Design review of the part built by this model. Coordinates are the model's own, in mm. A direction names the side the tool comes from. Coordinates: 2 decimals unless noted, no trailing zeros. Loops run counter-clockwise (first coordinate to the right, second up) from the corner with the lowest first, then second, coordinate; pieces in that order, holes last. Notation, with made-up numbers: (24.25, 73) -> (81.25, 73) arc R22 ccw to (81.25, 104) -> close; hole circle Ø10 at (22, 17). An arc over 180 degrees is marked (long way). One line per item, written item: value. Start each with the question number.
1. Add section C-C on z = 8.5. Write out the cut boundary in (x, y).
2. For probe 1 along X at (y, z) = (-72.5, 8.5); probe 2 along X at (y, z) = (-45.5, 58.5); probe 3 along X at (y, z) = (-45, 65), list the stretches that pass through material, from the lowest coordinate up.
3. Add section D-D on z = 55. Write out the cut boundary in (x, y), plus the area to 3 significant figures.
4. Draft analysis for pull direction X (two halves, no side actions). For faces 6 (the flat face through (-48.26, -76, 30)), 7 (the flat face through (-139, -67.31, 24)), 8 (the flat face through (157.48, -1, 24)), state which applies: pulls with the +X half, pulls with the -X half, needs draft (parallel to the pull), parting line crosses it, or undercut.
5. Insertion check: pin 1 (4 mm diameter, centred on y = -16.5, z = 70.5, fed in from +X); pin 2 (18 mm diameter, centred on x = -139, z = 17.5, fed in from +Y); pin 3 (8 mm diameter, centred on x = -105, y = 64, fed in from +Z). Each pin has a flat end and moves straight along its axis. Give the tip position at first contact, or say it passes through.
6. Add section A-A on x = -68.5. Write out the cut boundary in (y, z), plus the area to 3 significant figures.
7. Add section B-B on y = -22. Write out the cut boundary in (x, z).
8. Machinability: for faces 1 (the flat face through (-48.26, 75, 30)), 2 (the flat face through (140, 67.31, 24)), 3 (the flat face through (121.92, -1, 50)), 4 (the flat face through (-139, 67.31, 24)), 5 (the flat face through (-140, 1, 48.26)), which of the approach directions +Z, -Z, +X, -X, +Y, -Y give a long, thin tool a straight path to every point of the face, cutting with its end or side? Answer none if there is none.
```python
from build123d import *

# Parameters (mm, degrees)
F1_DEPTH   = 48.26
F2_W       = 35.56
F2_H       = 15.24
F3_DEPTH   = 25.4
F4_DEPTH   = 73.66
F5_START   = -73.66
F4_FACE_W  = 15.24
F4_FACE_H  = 25.4
F5_DEPTH   = 78.74
F6_DEPTH   = 22.86
F7_START   = 96.52
F6_FACE_W  = 15.24
F6_FACE_H  = 48.26
F7_DEPTH   = 73.66
F9_W       = 157.48
F9_H       = 67.31
F10_DEPTH  = 48.26
F11_W      = 35.56
F11_H      = 48.26
F12_DEPTH  = 16.51
F13_DEPTH  = 73.66
F14_START  = -73.66
F13_FACE_W = 16.51
F13_FACE_H = 48.26
F14_DEPTH  = 78.74
F18_DEPTH  = 12.7
F19_W      = 35.56
F19_H      = 134.62
F20_DEPTH  = 12.7
F22_DEPTH  = 13.97


with BuildPart() as f1:
    # F0 (on Top) → F1 (new body)
    with BuildSketch(Plane.XY):
        Polygon((0, 134.62), (0, 0), (314.96, 0), (314.96, 134.62), (35.56, 134.62), align=None)
    extrude(amount=F1_DEPTH)

    # F2 (on face) → F3 (join)
    with BuildSketch(Plane.XY.offset(48.26)):
        with Locations((17.78, 142.24)):
            Rectangle(F2_W, F2_H)
    extrude(amount=-F3_DEPTH)

    # F4 (add): a face of the model
    f4_faces = [f1.faces().sort_by_distance(p)[0] for p in [
        (35.56, 142.24, 35.56),
    ]]
    extrude(f4_faces, amount=F4_DEPTH)

    # F4_face (on face) → F5 (cut)
    with BuildSketch(Plane(origin=(109.22, 142.24, 35.56), x_dir=(0, 1, 0), z_dir=(1, 0, 0)).offset(F5_START)):
        Rectangle(F4_FACE_W, F4_FACE_H)
    extrude(amount=-F5_DEPTH, mode=Mode.SUBTRACT)

    # F6 (add): a face of the model
    f6_faces = [f1.faces().sort_by_distance(p)[0] for p in [
        (72.39, 142.24, 22.86),
    ]]
    extrude(f6_faces, amount=F6_DEPTH)

    # F6_face (on face) → F7 (join)
    with BuildSketch(Plane(origin=(109.22, 142.24, 24.13), x_dir=(0, 1, 0), z_dir=(1, 0, 0)).offset(F7_START)):
        Rectangle(F6_FACE_W, F6_FACE_H)
    extrude(amount=F7_DEPTH)


with BuildPart() as f10:
    # F9 (on Top) → F10 (new body)
    with BuildSketch(Plane.XY):
        with Locations((78.74, 33.655)):
            Rectangle(F9_W, F9_H)
    extrude(amount=F10_DEPTH)

    # F11 (on face) → F12 (join)
    with BuildSketch(Plane(origin=(0, 67.31, 0), x_dir=(-1, 0, 0), z_dir=(0, 1, 0))):
        with Locations((-139.7, 24.13)):
            Rectangle(F11_W, F11_H)
    extrude(amount=F12_DEPTH)

    # F13 (add): a face of the model
    f13_faces = [f10.faces().sort_by_distance(p)[0] for p in [
        (121.92, 75.565, 24.13),
    ]]
    extrude(f13_faces, amount=F13_DEPTH)

    # F13_face (on face) → F14 (cut)
    with BuildSketch(Plane(origin=(48.26, 75.565, 24.13), x_dir=(0, -1, 0), z_dir=(-1, 0, 0)).offset(F14_START)):
        Rectangle(F13_FACE_W, F13_FACE_H)
    extrude(amount=-F14_DEPTH, mode=Mode.SUBTRACT)

    # F15: F10 across plane


with BuildPart() as f10_1:
    add(f10.part)
    add(f10.part.mirror(Plane.XZ))

    # F16: F10 across plane


with BuildPart() as f10_2:
    add(f10_1.part)
    add(f10_1.part.mirror(Plane.YZ))

    # F17 (on face) → F18 (join)
    with BuildSketch(Plane.XY.offset(48.26)):
        Polygon((-121.92, 83.82), (-121.92, 67.31), (-121.92, -67.31), (-121.92, -83.82), (-48.26, -83.82), (-48.26, -67.31), (48.26, -67.31), (48.26, -83.82), (121.92, -83.82), (121.92, -67.31), (157.48, -67.31), (157.48, 67.31), (121.92, 67.31), (121.92, 83.82), (48.26, 83.82), (48.26, 67.31), (-48.26, 67.31), (-48.26, 83.82), align=None)
    extrude(amount=F18_DEPTH)

    # F19 (on face) → F20 (cut)
    with BuildSketch(Plane.XY.offset(60.96)):
        with Locations((139.7, 0)):
            Rectangle(F19_W, F19_H)
    extrude(amount=-F20_DEPTH, mode=Mode.SUBTRACT)

    # F21 (on face) → F22 (join)
    with BuildSketch(Plane.XY.offset(60.96)):
        Polygon((48.26, 67.31), (0, 67.31), (0, 0), (95.9053188562, 0), (95.9053188562, 67.31), align=None)
    extrude(amount=F22_DEPTH)

    # F23: F10 across plane


with BuildPart() as f10_3:
    add(f10_2.part)
    add(f10_2.part.mirror(Plane.XZ))

    # F24: F10 across plane


with BuildPart() as f10_4:
    add(f10_3.part)
    add(f10_3.part.mirror(Plane.YZ))


solid = f10_4.part
```
Worked answers:
1. outline: (-157.48, -67.31) -> (-121.92, -67.31) -> (-121.92, -83.82) -> (-48.26, -83.82) -> (-48.26, -67.31) -> (48.26, -67.31) -> (48.26, -83.82) -> (121.92, -83.82) -> (121.92, -67.31) -> (157.48, -67.31) -> (157.48, 67.31) -> (121.92, 67.31) -> (121.92, 83.82) -> (48.26, 83.82) -> (48.26, 67.31) -> (-48.26, 67.31) -> (-48.26, 83.82) -> (-121.92, 83.82) -> (-121.92, 67.31) -> (-157.48, 67.31) -> close
2. probe 1: x = -121.92 to -48.26, 48.26 to 121.92
2. probe 2: x = -121.92 to 121.92
2. probe 3: x = -95.91 to 95.91
3. outline: (-121.92, -83.82) -> (-48.26, -83.82) -> (-48.26, -67.31) -> (48.26, -67.31) -> (48.26, -83.82) -> (121.92, -83.82) -> (121.92, 83.82) -> (48.26, 83.82) -> (48.26, 67.31) -> (-48.26, 67.31) -> (-48.26, 83.82) -> (-121.92, 83.82) -> close
3. area: 37,700 mm²
4. face 6: undercut
4. face 7: needs draft
4. face 8: pulls with the +X half
5. pin 1: stops at x = 95.91
5. pin 2: stops at y = 67.31
5. pin 3: stops at z = 60.96
6. outline: (-83.82, 0) -> (83.82, 0) -> (83.82, 60.96) -> (67.31, 60.96) -> (67.31, 74.93) -> (-67.31, 74.93) -> (-67.31, 60.96) -> (-83.82, 60.96) -> close
6. area: 12,100 mm²
7. outline: (-157.48, 0) -> (157.48, 0) -> (157.48, 48.26) -> (121.92, 48.26) -> (121.92, 60.96) -> (95.91, 60.96) -> (95.91, 74.93) -> (-95.91, 74.93) -> (-95.91, 60.96) -> (-121.92, 60.96) -> (-121.92, 48.26) -> (-157.48, 48.26) -> close
8. face 1: +Z, -Z, +Y
8. face 2: +Z, -Z, +X, +Y
8. face 3: +Z, +X
8. face 4: +Z, -Z, -X, +Y
8. face 5: +Z, -X, +Y, -Y
